The listing builds one solid part. Answer for the finished solid, in the listing's coordinates (mm). A direction names the side the tool comes from. Round coordinates to 2 decimals unless told otherwise and drop trailing zeros. Order: outer loops, then holes, each group sorted by start corner. A loop starts at its lowest first (then second) coordinate and runs counter-clockwise, first axis right, second up. Notation, with made-up numbers: (-35, 66.5) - (-29, 66.5) arc R13 cw to (-29, 86.5) - close; hole circle Ø4 at (43.25, 72). An arc over 180 degrees is marked (long way). Write item = value, one per line.
from build123d import *

# Parameters (mm, degrees)
F1_DEPTH = 430
F2_R     = 4
F3_DEPTH = 30


with BuildPart() as f1:
    # F0 (on Right) → F1 (new body)
    with BuildSketch(Plane.YZ):
        with BuildLine():
            Line((12.5, 12.5), (-12.5, 12.5))
            ThreePointArc((-12.5, 12.5), (-21.338835, 8.838835), (-25, 0))
            ThreePointArc((-25, 0), (-21.338835, -8.838835), (-12.5, -12.5))
            Line((-12.5, -12.5), (12.5, -12.5))
            ThreePointArc((12.5, -12.5), (21.338835, -8.838835), (25, 0))
            ThreePointArc((25, 0), (21.338835, 8.838835), (12.5, 12.5))
        make_face()
        with BuildLine():
            Line((-12.5, 11), (12.5, 11))
            ThreePointArc((12.5, 11), (20.278175, 7.778175), (23.5, 0))
            ThreePointArc((23.5, 0), (20.278175, -7.778175), (12.5, -11))
            Line((12.5, -11), (-12.5, -11))
            ThreePointArc((-12.5, -11), (-20.278175, -7.778175), (-23.5, 0))
            ThreePointArc((-23.5, 0), (-20.278175, 7.778175), (-12.5, 11))
        make_face(mode=Mode.SUBTRACT)
    extrude(amount=-F1_DEPTH)

    # F2 (on face) → F3 (cut)
    with BuildSketch(Plane.XY.offset(12.5)):
        with Locations((-12.5, 0)):
            Circle(F2_R)
        with Locations((-417.5, 0)):
            Circle(F2_R)
    extrude(amount=-F3_DEPTH, mode=Mode.SUBTRACT)


solid = f1.part
Q1. Section A-A on y = 0 is taken. Determine the outline of the cut face in (x, z).
Model answer:
outline = (-430, -12.5) - (-421.5, -12.5) - (-421.5, -11) - (-430, -11) - close; (-430, 11) - (-421.5, 11) - (-421.5, 12.5) - (-430, 12.5) - close; (-413.5, -12.5) - (-16.5, -12.5) - (-16.5, -11) - (-413.5, -11) - close; (-413.5, 11) - (-16.5, 11) - (-16.5, 12.5) - (-413.5, 12.5) - close; (-8.5, -12.5) - (0, -12.5) - (0, -11) - (-8.5, -11) - close; (-8.5, 11) - (0, 11) - (0, 12.5) - (-8.5, 12.5) - close
Q2. Section B-B on x = -12.5 is taken. Determine the outline of the cut face in (y, z).
Model answer:
outline = (-25, 0) arc R12.5 ccw to (-12.5, -12.5) - (-4, -12.5) - (-4, -11) - (-12.5, -11) arc R11 cw to (-23.5, 0) arc R11 cw to (-12.5, 11) - (-4, 11) - (-4, 12.5) - (-12.5, 12.5) arc R12.5 ccw to start; (4, -12.5) - (12.5, -12.5) arc R12.5 ccw to (25, 0) arc R12.5 ccw to (12.5, 12.5) - (4, 12.5) - (4, 11) - (12.5, 11) arc R11 cw to (23.5, 0) arc R11 cw to (12.5, -11) - (4, -11) - close
Q3. Flat-ended cylindrical pins translate along their axes: P1, Ø12, axis at y = 5.5, z = -8.5, coming from the -X side; P2, Ø1, axis at x = -54, z = 6.5, coming from the -Y side; P3, Ø4, axis at x = -158, y = 16.5, coming from the -Z side; P4, Ø3, axis at x = -361.5, y = 16.5, coming from the +Z side. Find the tip coordinate at first contact, or state that the pin passes through.
Model answer:
P1 = -430
P2 = -23.47
P3 = -12.34
P4 = 12.25
Q4. Section D-D on z = -4.25 is taken. Determine the outline of the cut face in (x, y), then the cut area to 3 significant figures.
Model answer:
outline = (-430, -24.26) - (0, -24.26) - (0, -22.65) - (-430, -22.65) - close; (-430, 22.65) - (0, 22.65) - (0, 24.26) - (-430, 24.26) - close
area = 1,380 mm^2
Q5. Find the intervals of material crossed by line 1 (Z direction, x = -25.5, y = 11); line 2 (Y direction, x = -91, z = 1); line 3 (Y direction, x = -305, z = 7.5), in increasing order. Write a range as from..to.
Model answer:
line_1 = -12.5..-11, 11..12.5
line_2 = -24.96..-23.45, 23.45..24.96
line_3 = -22.5..-20.55, 20.55..22.5
Q6. For faces 4 (the face through (-15.7, -2.4, 11.8)), 5 (the face through (-212, 0, -11)), determine the directions among +Z, -Z, +X, -X, +Y, -Y from which every point of the face is accessible in a straight line to the end or side of a thin tool.
Model answer:
face_4 = +Z, -Z
face_5 = +X, -X
Q7. Section C-C on x = -327 is taken. Determine the outline of the cut face in (y, z).
Model answer:
outline = (-25, 0) arc R12.5 ccw to (-12.5, -12.5) - (12.5, -12.5) arc R12.5 ccw to (25, 0) arc R12.5 ccw to (12.5, 12.5) - (-12.5, 12.5) arc R12.5 ccw to start; hole (-23.5, 0) arc R11 ccw to (-12.5, -11) - (12.5, -11) arc R11 ccw to (23.5, 0) arc R11 ccw to (12.5, 11) - (-12.5, 11) arc R11 ccw to start
Q8. Determine the mould class of faces 1 (the face through (-15.7, -2.4, -11.7)), 2 (the face through (-212, 0, 12.5)), 3 (the face through (-430, -0.1, 11.2)) for opening direction X: released by +X, released by -X, zero draft, split by the parting line, or undercut.
Model answer:
face_1 = undercut
face_2 = zero draft
face_3 = released by -X
